Answer from the drawing. Dimensions are ordinates in mm from the lowest x, y and z of the part. Give positions to 0.01 mm unless a question says otherwise; leave off trailing zeros. Order: outer loops, then holes, each group sorted by start corner. A loop starts at its lowest first (then second) coordinate and runs counter-clockwise, first axis right, second up.
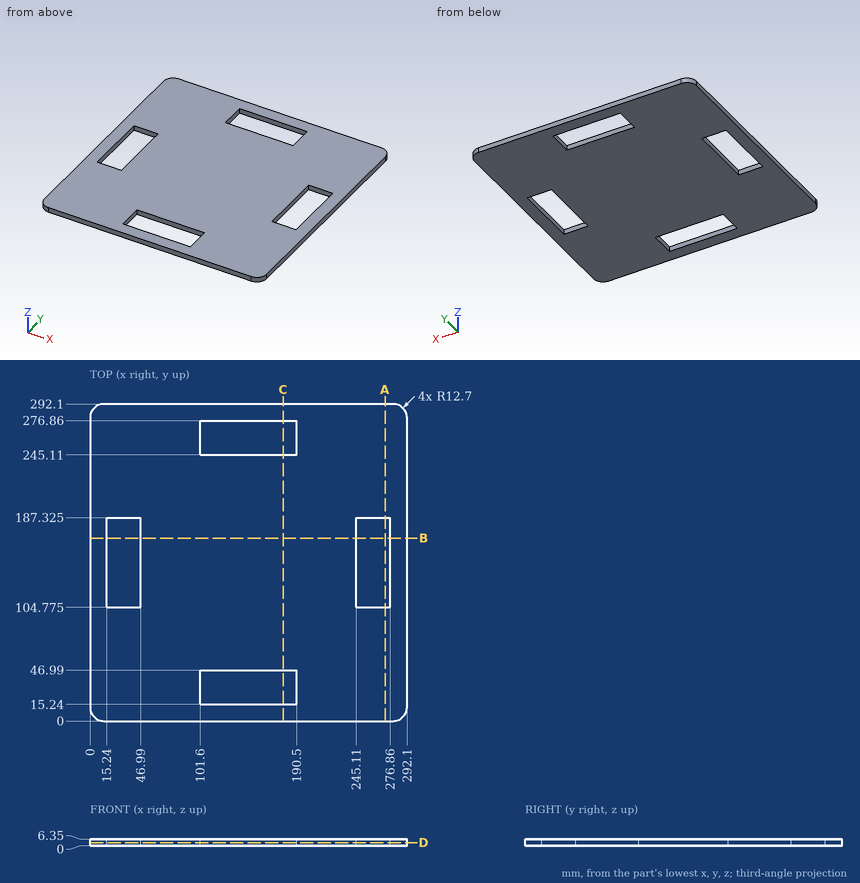
1. Straight lines are drawn through the part: probe 1 along Y at (x, z) = (145, 2); probe 2 along Y at (x, z) = (251, 4) (3 decimals). For each, find the intervals that lie inside material, in ascending order.
Findings below:
probe 1: y = 0 to 15.24, 46.99 to 245.11, 276.86 to 292.1
probe 2: y = 0 to 104.775, 187.325 to 292.1
2. The part is cut by section B-B (y = 168.5). Write down the section's boundary in (x, z).
Findings below:
outline: (0, 0) - (15.24, 0) - (15.24, 6.35) - (0, 6.35) - close; (46.99, 0) - (245.11, 0) - (245.11, 6.35) - (46.99, 6.35) - close; (276.86, 0) - (292.1, 0) - (292.1, 6.35) - (276.86, 6.35) - close
3. The part is cut by section D-D (z = 3). Write down the section's boundary in (x, y) (3 decimals).
Findings below:
outline: (0, 12.7) arc R12.7 ccw to (12.7, 0) - (279.4, 0) arc R12.7 ccw to (292.1, 12.7) - (292.1, 279.4) arc R12.7 ccw to (279.4, 292.1) - (12.7, 292.1) arc R12.7 ccw to (0, 279.4) - close; hole (15.24, 104.775) - (46.99, 104.775) - (46.99, 187.325) - (15.24, 187.325) - close; hole (101.6, 15.24) - (190.5, 15.24) - (190.5, 46.99) - (101.6, 46.99) - close; hole (101.6, 245.11) - (190.5, 245.11) - (190.5, 276.86) - (101.6, 276.86) - close; hole (245.11, 104.775) - (276.86, 104.775) - (276.86, 187.325) - (245.11, 187.325) - close
4. The part is cut by section A-A (x = 272). Write down the section's boundary in (y, z) (3 decimals).
Findings below:
outline: (0, 0) - (104.775, 0) - (104.775, 6.35) - (0, 6.35) - close; (187.325, 0) - (292.1, 0) - (292.1, 6.35) - (187.325, 6.35) - close
